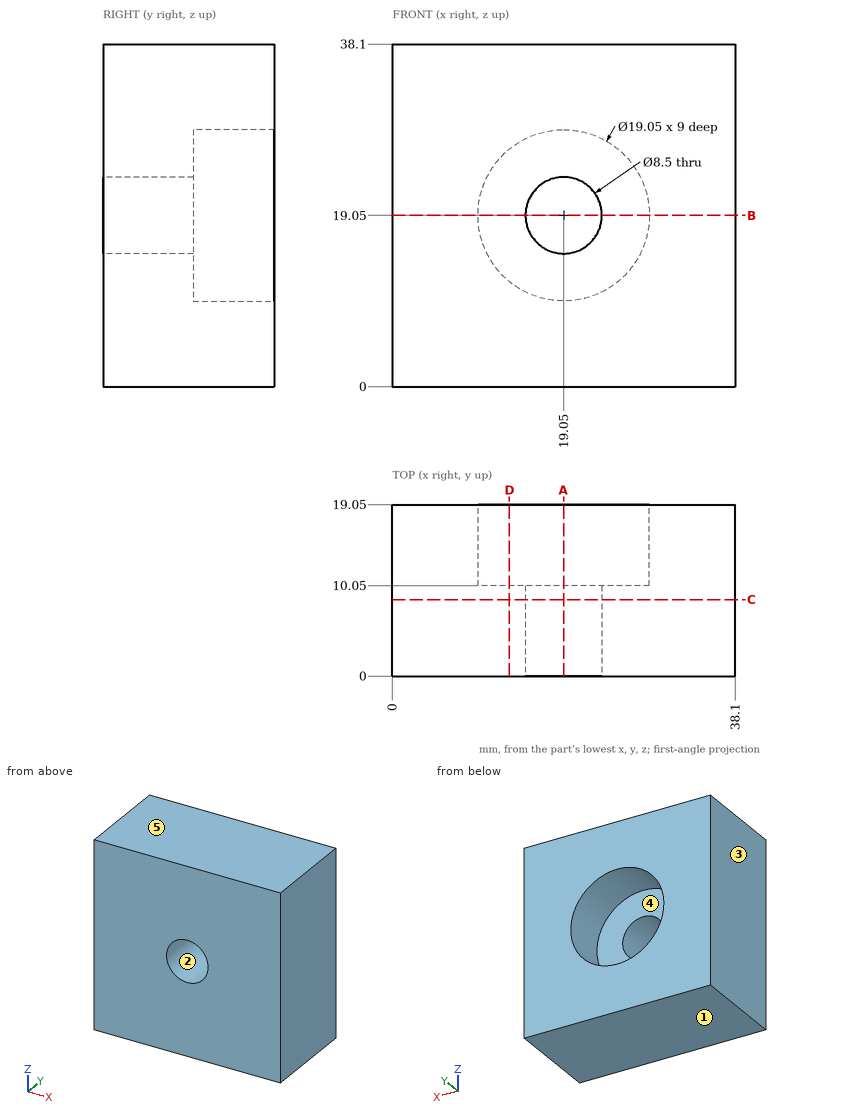
Input: dimensioned drawing with shaded views. Units: mm. Origin: part minimum x, y, z. A direction names the side the tool comes from. Coordinates: 2 decimals unless noted, no trailing zeros. Order: outer loops, then holes, each group sorted by start corner. A loop starts at its lowest first (then second) coordinate and runs counter-clockwise, first axis right, second up.
(1) Section query D-D (x = 13). Return the cut outline in (y, z).
(2) Section query B-B (z = 19.05). Return the cut outline in (x, y) (3 decimals), plus the area to 3 significant figures.
(3) Draft query along X for the marked faces 1, 2 and 3. Return one class per face: pulls with the +X half, pulls with the -X half, needs draft (parallel to the pull), parting line crosses it, or undercut.
(4) Section query C-C (y = 8.5). Return the cut outline in (x, z).
(5) First-contact query: pin 1 (13.5 mm diameter, centred on x = 19.05, z = 19.05, fed in from +Y). Flat tip, straight axial feed; report the tip coordinate or a pass-through.
(6) Section query A-A (x = 19.05). Return the cut outline in (y, z) (3 decimals), plus the area to 3 significant figures.
(7) Material intervals for probe 1 along X at (y, z) = (3.5, 19.05); probe 2 along X at (y, z) = (12.75, 19.05) (3 decimals), sorted ascending.
(8) Access query for the marked faces 4 and 5. Directions: +Z, -Z, +X, -X, +Y, -Y. A direction counts if a zero-diameter tool reaches every point of the face in a straight line with its end or side. Return the directions, or none.
Solution:
1. outline: (0, 0) - (19.05, 0) - (19.05, 11.69) - (10.05, 11.69) - (10.05, 26.41) - (19.05, 26.41) - (19.05, 38.1) - (0, 38.1) - close
2. outline: (0, 0) - (14.8, 0) - (14.8, 10.05) - (9.525, 10.05) - (9.525, 19.05) - (0, 19.05) - close; (23.3, 0) - (38.1, 0) - (38.1, 19.05) - (28.575, 19.05) - (28.575, 10.05) - (23.3, 10.05) - close
2. area: 469 mm2
3. face 1: needs draft
3. face 2: undercut
3. face 3: pulls with the -X half
4. outline: (0, 0) - (38.1, 0) - (38.1, 38.1) - (0, 38.1) - close; hole circle Ø8.5 at (19.05, 19.05)
5. pin 1: stops at y = 10.05
6. outline: (0, 0) - (19.05, 0) - (19.05, 9.525) - (10.05, 9.525) - (10.05, 14.8) - (0, 14.8) - close; (0, 23.3) - (10.05, 23.3) - (10.05, 28.575) - (19.05, 28.575) - (19.05, 38.1) - (0, 38.1) - close
6. area: 469 mm2
7. probe 1: x = 0 to 14.8, 23.3 to 38.1
7. probe 2: x = 0 to 9.525, 28.575 to 38.1
8. face 4: +Y
8. face 5: +Z, +X, -X, +Y, -Y
